Here's how the part is built. I have some questions about the finished solid (model axes, mm). Round coordinates to 2 decimals unless told otherwise and drop trailing zeros. Order: outer loops, then holes, each group sorted by start corner. A loop starts at its lowest first (then second) coordinate and runs counter-clockwise, first axis right, second up. Notation, with made-up numbers: (-30.5, -2) -> (0.5, -2) arc R18 cw to (0.5, 28) -> close; hole circle Ø5 at (-35, 15). An arc over 180 degrees is marked (long way). One line per item, written item: value.
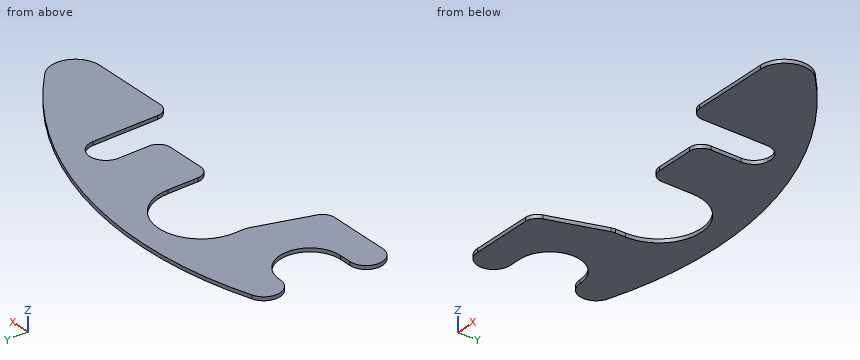
Autodesk Inventor part; units mm, degrees
ref_plane "YZ Plane" through (0, 0, 0) normal (1, 0, 0) x (0, 1, 0)
ref_plane "XZ Plane" through (0, 0, 0) normal (0, 1, 0) x (-1, 0, 0)
ref_plane "XY Plane" through (0, 0, 0) normal (0, 0, 1) x (1, 0, 0)
sketch "Sketch1" plane through (0, 0, 0) normal (0, 0, 1) x (1, 0, 0)
  circle A0 centre (0, 0) radius 3.5
  circle A1 centre (10, 0) radius 1.35
  circle A2 centre (18.7217, -4.35) radius 2
  line L0 (-3.5, 0) -> (-3.5, -1)
  line L1 (-3.5, -1) -> (-5.2383, -6.35)
  line L2 (-5.2383, -6.35) -> (-11, -6.35)
  line L3 (3.5, 0) -> (3.5, -3.5)
  line L4 (3.5, -3.5) -> (8.65, -3.5)
  line L5 (8.65, -3.5) -> (8.65, 0)
  arc A3 (20.1001, -2.9009) -> (-10.4205, 3.9828) centre (-0.9208, -25) ccw
  circle A4 centre (-10, 2.7) radius 1.35
  circle A5 centre (-11, -5) radius 1.35
  line L6 (18.7217, -6.35) -> (11.35, -6.35)
  line L7 (11.35, -6.35) -> (11.35, 0)
  line L8 (-11, -3.65) -> (-10, -3.65)
  arc A6 (-10, -3.65) -> (-10, 1.35) centre (-10, -1.15) ccw
  line L9 (-10, 1.35) -> (-10, 1.35)
  dimension "d0" = 3.5
  dimension "d1" = 1.35
  dimension "d2" = 10
  dimension "d5" = 1
  dimension "d6" = 30.5
  dimension "d10" = 20
  dimension "d15" = 21.5
  dimension "d16" = 18
  dimension "d18" = 2
  dimension "d20" = 10
  dimension "d21" = 11
  dimension "d22" = 2.5
extrude "Extrusion1" add sketch "Sketch1" along normal blind 0.3 contours A0 L0 L1 L2 A5 L8 A6 A4 A3 A2 L6 L7 A1 L5 L4 L3 | A5 | A2 | A4
fillet "Fillet1" radius 1 5 edges at (-5.2383, -6.35, 0.15) (-3.5, -1, 0.15) (3.5, -3.5, 0.15) (8.65, -3.5, 0.15) (11.35, -6.35, 0.15)
properties part number "308-15" material "Steel"
Q1. I need wall thicknesses on line 1 along X through (y, z) = (-2.25, 0.1) (3 decimals); line 2 along X through (y, z) = (1, 0.2); line 3 along X through (y, z) = (2.75, 0.1). Which ranges of each line are inside material? Lowest first, please.
Answers:
line 1: -7.755 to -3.906, 3.5 to 8.65, 11.35 to 19.394
line 2: -8.72 to -3.35, 3.35 to 9.09, 10.91 to 15.02
line 3: -11.35 to -2.17, 2.17 to 11.74
Q2. I want a section at B-B on z = 0.2. Write out the boundary of the cut face in (x, y).
Answers:
outline: (-11, -6.35) -> (-5.96, -6.35) arc R1 ccw to (-5.01, -5.66) -> (-3.55, -1.15) arc R1 ccw to (-3.5, -0.84) -> (-3.5, 0) arc R3.5 cw to (3.5, 0) -> (3.5, -2.5) arc R1 ccw to (4.5, -3.5) -> (7.65, -3.5) arc R1 ccw to (8.65, -2.5) -> (8.65, 0) arc R1.35 cw to (11.35, 0) -> (11.35, -5.35) arc R1 ccw to (12.35, -6.35) -> (18.72, -6.35) arc R2 ccw to (20.1, -2.9) arc R30.5 ccw to (-10.42, 3.98) arc R1.35 ccw to (-10, 1.35) arc R2.5 cw to (-10, -3.65) -> (-11, -3.65) arc R1.35 ccw to start
Q3. I want a section at A-A on y = 2.75. Write out the boundary of the cut face in (x, z).
Answers:
outline: (-11.35, 0) -> (-2.17, 0) -> (-2.17, 0.3) -> (-11.35, 0.3) -> close; (2.17, 0) -> (11.74, 0) -> (11.74, 0.3) -> (2.17, 0.3) -> close
Q4. I want a section at D-D on x = 13.5. Write out the boundary of the cut face in (y, z), then the cut area to 3 significant figures.
Answers:
outline: (-6.35, 0) -> (1.88, 0) -> (1.88, 0.3) -> (-6.35, 0.3) -> close
area: 2.47 mm2
Q5. I want a section at C-C on x = 0. Write out the boundary of the cut face in (y, z), then the cut area to 3 significant figures.
Answers:
outline: (3.5, 0) -> (5.49, 0) -> (5.49, 0.3) -> (3.5, 0.3) -> close
area: 0.596 mm2
